Autodesk Inventor part; units mm, degrees
ref_plane "YZ Plane" through (0, 0, 0) normal (1, 0, 0) x (0, 1, 0)
ref_plane "XZ Plane" through (0, 0, 0) normal (0, 1, 0) x (-1, 0, 0)
ref_plane "XY Plane" through (0, 0, 0) normal (0, 0, 1) x (1, 0, 0)
sketch "Sketch1" plane through (0, 0, 0) normal (0, 1, 0) x (-1, 0, 0)
  arc A0 (-152, 0) -> (152, 0) centre (0, 100) ccw
  line L0 (0, -81.945) -> (-47.311, 0)
  line L1 (-47.311, 0) -> (47.311, 0) construction
  line L2 (47.311, 0) -> (0, -81.945)
  line L3 (0, 0) -> (68.5411, -68.5411)
  line L4 (0, 0) -> (-68.5411, -68.5411)
  line L5 (47.311, 0) -> (116.3651, -39.8684)
  line L6 (-47.311, 0) -> (-116.3651, -39.8684)
  line L7 (114.7776, -42.618) -> (48.4731, -4.3371)
  line L8 (48.4731, -4.3371) -> (0, -88.295)
  line L9 (0, -88.295) -> (-48.4731, -4.3371)
  line L10 (-48.4731, -4.3371) -> (-114.4332, -42.4192)
  line L11 (-66.0999, -70.5901) -> (0, -4.4901)
  line L12 (0, -4.4901) -> (66.2961, -70.7862)
  line L13 (116.3651, -39.8684) -> (114.7776, -42.618)
  line L14 (68.5411, -68.5411) -> (66.2961, -70.7862)
  line L15 (-66.0999, -70.5901) -> (-67.8825, -68.8075)
  line L16 (-114.4332, -42.4192) -> (-115.4867, -40.5945)
  arc A1 (-157.2837, -3.5223) -> (157.2837, -3.5223) centre (0, 100) ccw
  line L17 (157.2837, -3.5223) -> (152, 0)
  line L18 (-152, 0) -> (-157.2837, -3.5223)
  line L19 (116.3651, -39.8684) -> (113.3651, -39.8684)
  line L20 (113.3651, -39.8684) -> (113.3651, 0)
  line L21 (113.3651, 0) -> (116.3651, 0)
  line L22 (116.3651, 0) -> (116.3651, -39.8684)
  line L23 (0, 0) -> (0, -27.315) construction
  line L24 (-116.3651, -39.8684) -> (-113.3651, -39.8684)
  line L25 (-113.3651, -39.8684) -> (-113.3651, 0)
  line L26 (-113.3651, 0) -> (-116.3651, 0)
  line L27 (-116.3651, 0) -> (-116.3651, -39.8684)
  point P0 (-3.6878, -81.9077)
  point P1 (-65.3239, -69.814)
  point P2 (-30.6747, -35.1649)
  point P3 (29.994, -29.994)
  point P4 (-29.994, -29.994)
  point P5 (32.3182, -32.3182)
  point P6 (113.7344, -42.0158)
  point P7 (30.6747, -35.1649)
  point P8 (65.3239, -69.814)
  point P9 (3.6878, -81.9077)
  point P10 (-28.3505, -32.8406)
  point P11 (28.3505, -32.8406)
  point P12 (-32.3182, -32.3182)
  point P13 (-113.7344, -42.0158)
  point P14 (-113.3651, -38.1363)
  point P15 (113.3651, -38.1363)
  point P16 (0, 0)
  dimension "d0" = 152
  dimension "d1" = 152
  dimension "d2" = 100
  dimension "d3" = 0
  dimension "d4" = 45
  dimension "d8" = 3.175
  dimension "d9" = 3.175
  dimension "d10" = 6.35
  dimension "d11" = 6.35
  dimension "d12" = 3.5223
  dimension "d13" = 3.5223
  dimension "d29" = 3
  dimension "d30" = 157.2837
extrude "Extrusion1" add sketch "Sketch1" along normal mid plane 3 contours A0 L16 L10 L15 L11 L9 A1 L18 | L24 L25 L6 L0 L4 L9 L10 A0 | L27 L26 L25 L6 | L6 L25 L24 | A0 L10 L16 | L9 A0 L8 | L8 A0 L12 L14 L7 L13 L17 A1 | A0 L2 L12 L8 | L9 L11 L0 A0 | L4 L9 L11 A0 | L4 L3 L2 L12 L11 L0 | L0 L11 L9 L4 | L12 L8 L3 A0 | A0 L14 L12 | L12 L2 L3 L8 | L11 L15 A0 | L3 L2 L5 L20 L19 A0 L7 L8 | L13 L7 A0 | L19 L20 L5 | L5 L20 L21 L22
sketch "Sketch2" plane through (0, 1.5, 0) normal (0, 1, 0) x (1, 0, 0)
  line L0 (0, 0) -> (29.994, 29.994)
  line L1 (0, 0) -> (200, 0)
  line L2 (200, 0) -> (200, 200)
  line L3 (200, 200) -> (0, 200)
  line L4 (0, 200) -> (0, 0)
  dimension "d16" = 200
  dimension "d17" = 200
extrude "Extrusion2" cut sketch "Sketch2" along normal through all both and the other way through all
sketch "Sketch3" plane through (0, 1.5, 0) normal (0, 1, 0) x (1, 0, 0)
  line L0 (-29.994, 29.994) -> (0, 0)
  circle A0 centre (0, 0) radius 5
  line L1 (-157.2837, 3.5223) -> (-152, 0)
  line L2 (-47.311, 0) -> (-29.994, 29.994)
  circle A1 centre (-47.311, 0) radius 5
  line L3 (0, 81.945) -> (0, 88.295)
  circle A2 centre (0, 85.12) radius 5
  circle A3 centre (-152, 0) radius 5
  line L4 (-116.3651, 0) -> (-113.3651, 0)
  circle A4 centre (-114.8651, 0) radius 5
  dimension "d20" = 10
extrude "Circular_Mounts" add sketch "Sketch3" against normal blind 3
sketch "Sketch4" plane through (0, 1.5, 0) normal (0, 1, 0) x (1, 0, 0)
  arc A0 (-51.6411, 2.5) -> (-44.811, 4.3301) centre (-47.311, 0) ccw
  circle A1 centre (-47.311, 0) radius 4.05
  circle A2 centre (0, 0) radius 4.05
  arc A3 (-156.1603, 2.7735) -> (-149.1948, 4.1389) centre (-152, 0) ccw
  circle A4 centre (-152, 0) radius 4.05
  arc A5 (-0.9958, 80.2202) -> (-3.8953, 88.2548) centre (0, 85.12) ccw
  circle A6 centre (0, 85.12) radius 4.05
  arc A7 (-116.3651, 4.7697) -> (-113.3651, 4.7697) centre (-114.8651, 0) ccw
  circle A8 centre (-114.8651, 0) radius 4.05
  dimension "d23" = 8.1
extrude "Inserts" add sketch "Sketch4" along normal blind 4
fillet "Fillet2" radius 0.5 5 edges at (-156.05, 5.5, 0) (-51.361, 5.5, 0) (-4.05, 5.5, 0) (-4.05, 5.5, -85.12) (-118.9151, 5.5, 0)
fillet "Fillet3" radius 2 2 edges at (-156.1603, 0, -2.7735) (-157.2837, 0, -3.5223)
equation "\"d1\" = d0"
properties part number "W-Support" material "ABS Plastic"
Here's how the part is built. I have some questions about the finished solid (model axes, mm). A direction names the side the tool comes from. Give positions to 0.01 mm unless a question says otherwise; leave off trailing zeros. Order: outer loops, then holes, each group sorted by start corner. A loop starts at its lowest first (then second) coordinate and runs counter-clockwise, first axis right, second up. Notation, with made-up numbers: M -0.75,76 L 47.25,76 A33 ccw 47.25,105 Z; hole C 51,22.25 d5. An arc over 180 degrees is marked long. Use a Markdown table: item, result. Add a question column.
1. Suppose I cut it at B-B (z = -11). List the corners of the cut face in (x, y) for me, and give its area (3 significant figures).
2. Suppose I cut it at C-C (x = -18). List the corners of the cut face in (y, z) for me, and give its area (3 significant figures).
3. For pin 1 Ø3.5 at (y, z) = (-0.5, -14) entering from -X; pin 2 Ø3.5 at (y, z) = (-0.5, -17.5) entering from +X; pin 3 Ø3 at (x, y) = (-131, -0.5) entering from -Z, each with a flat end and sliding along its axis, tell me the tip position at first contact or that it passes through.
4. On a 3-axis mill with a long thin cutter (end or side, diameter ignored), from which of +Z, -Z, +X, -X, +Y, -Y can I reach the whole of each face in a straight line? I mean faces 1 (the flat face through (-17.4, -0.02, -58.16)), 2 (the flat face through (0, 5.5, -85)), 3 (the flat face through (-14.22, -0.02, -18.71)), 4 (the cylindrical face through (-0.878, 3.226, -3.954)). Say none if no direction works.
5. If we mould it in two halves opening along Z, with no side actions, what happens to faces 5 (the flat face through (-81.854, -0.021, -23.61)), 6 (the cylindrical face through (-91.603, -0.021, -64.511)), 7 (the flat face through (0, 5.5, 0))? For each: +Z half, -Z half, draft (parallel to the pull), parting line (faces both ways), or undercut.
6. Suppose I cut it at A-A (x = -88.5). List the corners of the cut face in (y, z) for me.
7. I need wall thicknesses on probe 1 along X at (y, z) = (3.5, -2); probe 2 along X at (y, z) = (-0.5, -0.5); probe 3 along Z at (x, y) = (-41.5, 1.25). Which ranges of each line are inside material? Lowest first, please. Write a range as from..to.
8. Suppose I cut it at D-D (y = -0.25). List the corners of the cut face in (x, z) for me, and give its area (3 significant figures).
Results list:
| question | item | result |
|---|---|---|
| 1 | outline | M -152.1,-1.5 L -144.16,-1.5 L -144.16,1.5 L -152.1,1.5 Z; M -116.37,-1.5 L -113.37,-1.5 L -113.37,1.5 L -116.37,1.5 Z; M -66.36,-1.5 L -60.01,-1.5 L -60.01,1.5 L -66.36,1.5 Z; M -44.63,-1.5 L -40.96,-1.5 L -40.96,1.5 L -44.63,1.5 Z; M -11,-1.5 L -6.51,-1.5 L -6.51,1.5 L -11,1.5 Z |
| 1 | area | 76.3 mm² |
| 2 | outline | M -1.5,-87.43 L 1.5,-87.43 L 1.5,-81.05 L -1.5,-81.05 Z; M -1.5,-57.12 L 1.5,-57.12 L 1.5,-50.77 L -1.5,-50.77 Z; M -1.5,-22.49 L 1.5,-22.49 L 1.5,-18 L -1.5,-18 Z |
| 2 | area | 51.7 mm² |
| 3 | pin 1 | stops at x = -151.18 |
| 3 | pin 2 | stops at x = -11.26 |
| 3 | pin 3 | stops at z = -36.69 |
| 4 | face 1 | +Y, -Y |
| 4 | face 2 | +Z, -Z, +X, -X, +Y |
| 4 | face 3 | +X, +Y, -Y |
| 4 | face 4 | +Y |
| 5 | face 5 | undercut |
| 5 | face 6 | -Z half |
| 5 | face 7 | draft |
| 6 | outline | M -1.5,-66.2 L 1.5,-66.2 L 1.5,-58.97 L -1.5,-58.97 Z; M -1.5,-27.45 L 1.5,-27.45 L 1.5,-23.78 L -1.5,-23.78 Z |
| 7 | probe 1 | x = -155.52..-148.48, -118.39..-111.34, -50.83..-43.79, -3.52..3.52 |
| 7 | probe 2 | x = -156.97..-147.03, -119.84..-109.89, -52.29..-42.34, -4.97..4.97 |
| 7 | probe 3 | z = -83.66..-77.15, -45.99..-41.5, -16.41..-10.06 |
| 8 | outline | M -156.8,-2.78 A2 ccw -156.59,-4.57 A188.3 ccw -3.9,-88.25 A5 ccw long -1,-80.22 L -28.35,-32.84 L -0.49,-4.98 A5 ccw long -3.54,-3.54 L -29.99,-29.99 L -44.81,-4.33 A5 ccw long -51.64,-2.5 L -113.37,-38.14 L -113.37,-4.77 A5 ccw long -116.37,-4.77 L -116.37,-39.87 A181.95 cw -149.19,-4.14 A5 ccw long -156.77,-1.49 A2 cw Z; hole M -113.73,-42.02 A181.95 ccw -68.54,-68.54 L -32.32,-32.32 L -48.13,-4.93 A5 cw -49.07,-4.68 Z; hole M -65.32,-69.81 A181.95 ccw -3.83,-81.9 A5 cw -3.75,-81.81 L -30.67,-35.16 Z |
| 8 | area | 2,400 mm² |
